```python
from build123d import *

# Parameters (mm, degrees)
SKETCH_1_R      = 3.1
SKETCH_1_R_2    = 2.05
EXTRUDE_2_DEPTH = 2
FILLET_1_R      = 1.3


with BuildPart() as part:
    # 草图1 → 凸台-拉伸2 (new body)
    with BuildSketch(Plane.XY):
        with BuildLine():
            Line((26.037512023, -61.503506411), (-55.962487977, -61.503506411))
            Line((-55.962487977, -61.503506411), (-55.962487977, -56.053506411))
            Line((-55.962487977, -56.053506411), (-51.962487977, -56.053506411))
            Line((-51.962487977, -56.053506411), (-51.962487977, -57.503506411))
            Line((-51.962487977, -57.503506411), (-48.762487977, -57.503506411))
            Line((-48.762487977, -57.503506411), (-48.762487977, -56.053506411))
            Line((-48.762487977, -56.053506411), (-45.562487977, -56.053506411))
            Line((-45.562487977, -56.053506411), (-45.562487977, -51.953506411))
            Line((-45.562487977, -51.953506411), (-48.762487977, -51.953506411))
            Line((-48.762487977, -51.953506411), (-48.762487977, -50.503506411))
            Line((-48.762487977, -50.503506411), (-51.962487977, -50.503506411))
            Line((-51.962487977, -50.503506411), (-51.962487977, -51.953506411))
            Line((-51.962487977, -51.953506411), (-55.962487977, -51.953506411))
            Line((-55.962487977, -51.953506411), (-55.962487977, -43.003506411))
            Line((-55.962487977, -43.003506411), (-60.962487977, -43.003506411))
            Line((-60.962487977, -43.003506411), (-60.962487977, -35.003506411))
            Line((-60.962487977, -35.003506411), (-55.962487977, -35.003506411))
            Line((-55.962487977, -35.003506411), (-55.962487977, -26.053506411))
            Line((-55.962487977, -26.053506411), (-51.962487977, -26.053506411))
            Line((-51.962487977, -26.053506411), (-51.962487977, -27.503506411))
            Line((-51.962487977, -27.503506411), (-48.762487977, -27.503506411))
            Line((-48.762487977, -27.503506411), (-48.762487977, -26.053506411))
            Line((-48.762487977, -26.053506411), (-45.562487977, -26.053506411))
            Line((-45.562487977, -26.053506411), (-45.562487977, -21.953506411))
            Line((-45.562487977, -21.953506411), (-48.762487977, -21.953506411))
            Line((-48.762487977, -21.953506411), (-48.762487977, -20.503506411))
            Line((-48.762487977, -20.503506411), (-51.962487977, -20.503506411))
            Line((-51.962487977, -20.503506411), (-51.962487977, -21.953506411))
            Line((-51.962487977, -21.953506411), (-55.962487977, -21.953506411))
            Line((-55.962487977, -21.953506411), (-55.962487977, -13.003506411))
            Line((-55.962487977, -13.003506411), (-60.962487977, -13.003506411))
            Line((-60.962487977, -13.003506411), (-60.962487977, -5.003506411))
            Line((-60.962487977, -5.003506411), (-55.962487977, -5.003506411))
            Line((-55.962487977, -5.003506411), (-55.962487977, 3.946493589))
            Line((-55.962487977, 3.946493589), (-51.962487977, 3.946493589))
            Line((-51.962487977, 3.946493589), (-51.962487977, 2.496493589))
            Line((-51.962487977, 2.496493589), (-48.762487977, 2.496493589))
            Line((-48.762487977, 2.496493589), (-48.762487977, 3.946493589))
            Line((-48.762487977, 3.946493589), (-45.562487977, 3.946493589))
            Line((-45.562487977, 3.946493589), (-45.562487977, 8.046493589))
            Line((-45.562487977, 8.046493589), (-48.762487977, 8.046493589))
            Line((-48.762487977, 8.046493589), (-48.762487977, 9.496493589))
            Line((-48.762487977, 9.496493589), (-51.962487977, 9.496493589))
            Line((-51.962487977, 9.496493589), (-51.962487977, 8.046493589))
            Line((-51.962487977, 8.046493589), (-55.962487977, 8.046493589))
            Line((-55.962487977, 8.046493589), (-55.962487977, 23.496493589))
            Line((-55.962487977, 23.496493589), (-55.962487977, 31.722989041))
            ThreePointArc((-55.962487977, 31.722989041), (-14.962487977, 51.269592797), (26.037512023, 31.722989041))
            Line((26.037512023, 31.722989041), (26.037512023, 23.496493589))
            Line((26.037512023, 23.496493589), (26.037512023, 8.046493589))
            Line((26.037512023, 8.046493589), (22.037512023, 8.046493589))
            Line((22.037512023, 8.046493589), (22.037512023, 9.496493589))
            Line((22.037512023, 9.496493589), (18.837512023, 9.496493589))
            Line((18.837512023, 9.496493589), (18.837512023, 8.046493589))
            Line((18.837512023, 8.046493589), (15.637512023, 8.046493589))
            Line((15.637512023, 8.046493589), (15.637512023, 3.946493589))
            Line((15.637512023, 3.946493589), (18.837512023, 3.946493589))
            Line((18.837512023, 3.946493589), (18.837512023, 2.496493589))
            Line((18.837512023, 2.496493589), (22.037512023, 2.496493589))
            Line((22.037512023, 2.496493589), (22.037512023, 3.946493589))
            Line((22.037512023, 3.946493589), (26.037512023, 3.946493589))
            Line((26.037512023, 3.946493589), (26.037512023, -5.003506411))
            Line((26.037512023, -5.003506411), (31.037512023, -5.003506411))
            Line((31.037512023, -5.003506411), (31.037512023, -13.003506411))
            Line((31.037512023, -13.003506411), (26.037512023, -13.003506411))
            Line((26.037512023, -13.003506411), (26.037512023, -21.953506411))
            Line((26.037512023, -21.953506411), (22.037512023, -21.953506411))
            Line((22.037512023, -21.953506411), (22.037512023, -20.503506411))
            Line((22.037512023, -20.503506411), (18.837512023, -20.503506411))
            Line((18.837512023, -20.503506411), (18.837512023, -21.953506411))
            Line((18.837512023, -21.953506411), (15.637512023, -21.953506411))
            Line((15.637512023, -21.953506411), (15.637512023, -26.053506411))
            Line((15.637512023, -26.053506411), (18.837512023, -26.053506411))
            Line((18.837512023, -26.053506411), (18.837512023, -27.503506411))
            Line((18.837512023, -27.503506411), (22.037512023, -27.503506411))
            Line((22.037512023, -27.503506411), (22.037512023, -26.053506411))
            Line((22.037512023, -26.053506411), (26.037512023, -26.053506411))
            Line((26.037512023, -26.053506411), (26.037512023, -35.003506411))
            Line((26.037512023, -35.003506411), (31.037512023, -35.003506411))
            Line((31.037512023, -35.003506411), (31.037512023, -43.003506411))
            Line((31.037512023, -43.003506411), (26.037512023, -43.003506411))
            Line((26.037512023, -43.003506411), (26.037512023, -51.953506411))
            Line((26.037512023, -51.953506411), (22.037512023, -51.953506411))
            Line((22.037512023, -51.953506411), (22.037512023, -50.503506411))
            Line((22.037512023, -50.503506411), (18.837512023, -50.503506411))
            Line((18.837512023, -50.503506411), (18.837512023, -51.953506411))
            Line((18.837512023, -51.953506411), (15.637512023, -51.953506411))
            Line((15.637512023, -51.953506411), (15.637512023, -56.053506411))
            Line((15.637512023, -56.053506411), (18.837512023, -56.053506411))
            Line((18.837512023, -56.053506411), (18.837512023, -57.503506411))
            Line((18.837512023, -57.503506411), (22.037512023, -57.503506411))
            Line((22.037512023, -57.503506411), (22.037512023, -56.053506411))
            Line((22.037512023, -56.053506411), (26.037512023, -56.053506411))
            Line((26.037512023, -56.053506411), (26.037512023, -61.503506411))
        make_face()
        with Locations((-14.962487977, -25.253506411)):
            Circle(SKETCH_1_R, mode=Mode.SUBTRACT)
        with Locations((4.523083608, -12.753506411)):
            Circle(SKETCH_1_R, mode=Mode.SUBTRACT)
        with Locations((-14.962487977, -1.503506411)):
            Circle(SKETCH_1_R_2, mode=Mode.SUBTRACT)
        with Locations((-35.530591317, 10.371493589)):
            Circle(SKETCH_1_R, mode=Mode.SUBTRACT)
        with Locations((-34.448059562, -12.753506411)):
            Circle(SKETCH_1_R, mode=Mode.SUBTRACT)
        with Locations((5.605615363, 10.371493589)):
            Circle(SKETCH_1_R, mode=Mode.SUBTRACT)
        with Locations((-14.962487977, 20.996493589)):
            Circle(SKETCH_1_R, mode=Mode.SUBTRACT)
        with Locations((18.271530739, -34.737525127)):
            Circle(SKETCH_1_R_2, mode=Mode.SUBTRACT)
        with Locations((-14.962487977, -48.503506411)):
            Circle(SKETCH_1_R_2, mode=Mode.SUBTRACT)
        with Locations((-48.196506692, -34.737525127)):
            Circle(SKETCH_1_R_2, mode=Mode.SUBTRACT)
        with Locations((-48.196506692, 31.730512305)):
            Circle(SKETCH_1_R_2, mode=Mode.SUBTRACT)
        with Locations((-14.962487977, 45.496493589)):
            Circle(SKETCH_1_R_2, mode=Mode.SUBTRACT)
        with Locations((18.271530739, 31.730512305)):
            Circle(SKETCH_1_R_2, mode=Mode.SUBTRACT)
    extrude(amount=EXTRUDE_2_DEPTH)

    # 圆角1
    fillet_1_edges = [part.edges().sort_by_distance(p)[0] for p in [
        (-60.962487977, -43.003506411, 1),
        (-60.962487977, -35.003506411, 1),
        (-60.962487977, -13.003506411, 1),
        (-60.962487977, -5.003506411, 1),
        (31.037512023, -5.003506411, 1),
        (31.037512023, -13.003506411, 1),
        (31.037512023, -35.003506411, 1),
        (31.037512023, -43.003506411, 1),
    ]]
    fillet(fillet_1_edges, radius=FILLET_1_R)


solid = part.part
```
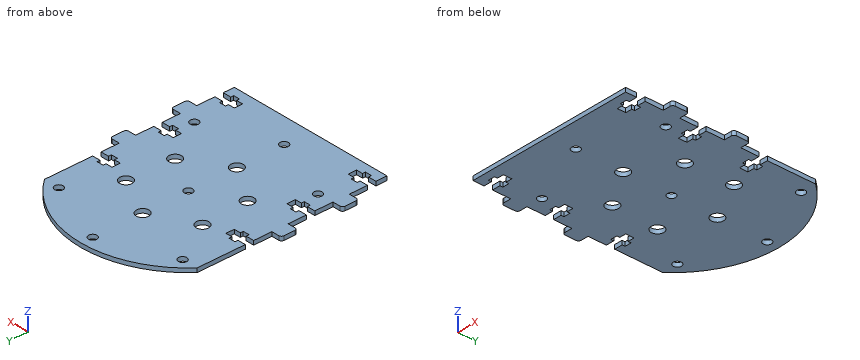
Work out the finished part from the listing and answer in its coordinate system (mm). Coordinates: 2 decimals unless noted, no trailing zeros. Order: outer loops, then holes, each group sorted by start corner. A loop starts at its lowest first (then second) coordinate and runs counter-clockwise, first axis right, second up. Notation, with made-up numbers: (24.5, 87) - (57.5, 87) arc R16 ccw to (57.5, 103) - close; hole circle Ø5 at (-13, 54). An arc over 180 degrees is marked (long way). Answer as a JSON object with one key per item and string values.
1. Find section C-C on z = 0.6. Count the separate pieces of the cut face and the enclosed holes in it, plus the area to 3 significant figures.
Output values:
{"separate pieces": "1", "enclosed holes": "13", "area": "8,330 mm²"}
2. Consider line 1 (Y direction, x = 22.5, z = 1.25); line 2 (Y direction, x = -34, z = 0.6); line 3 (Y direction, x = -15.5, z = 0.25). Determine where each line is inside the solid, lowest interval first.
Output values:
{"line 1": "y = -61.5 to -56.05, -51.95 to -26.05, -21.95 to 3.95, 8.05 to 35.67", "line 2": "y = -61.5 to -15.82, -9.69 to 7.68, 13.07 to 47.72", "line 3": "y = -61.5 to -50.48, -46.53 to -28.31, -22.2 to -3.48, 0.47 to 17.94, 24.05 to 43.52, 47.47 to 51.27"}
3. Find section A-A on x = 23.5. Determine the outline of the cut face in (y, z).
Output values:
{"outline": "(-61.5, 0) - (-56.05, 0) - (-56.05, 2) - (-61.5, 2) - close; (-51.95, 0) - (-26.05, 0) - (-26.05, 2) - (-51.95, 2) - close; (-21.95, 0) - (3.95, 0) - (3.95, 2) - (-21.95, 2) - close; (8.05, 0) - (34.63, 0) - (34.63, 2) - (8.05, 2) - close"}
4. Each of these flat-tipped pins is pushed along its axis until it touches: P1, Ø1, axis at x = 28, z = 1, coming from the -Y side; P2, Ø1.2, axis at y = -21, z = 0.5, coming from the -X side. Where does it stop, or does it pass through?
Output values:
{"P1": "stops at y = -43", "P2": "stops at x = -55.96"}
5. Find section B-B on x = -47.5. Determine the outline of the cut face in (y, z).
Output values:
{"outline": "(-61.5, 0) - (-56.05, 0) - (-56.05, 2) - (-61.5, 2) - close; (-51.95, 0) - (-36.67, 0) - (-36.67, 2) - (-51.95, 2) - close; (-32.81, 0) - (-26.05, 0) - (-26.05, 2) - (-32.81, 2) - close; (-21.95, 0) - (3.95, 0) - (3.95, 2) - (-21.95, 2) - close; (8.05, 0) - (29.8, 0) - (29.8, 2) - (8.05, 2) - close; (33.66, 0) - (40.05, 0) - (40.05, 2) - (33.66, 2) - close"}
